from build123d import *

# Parameters (mm, degrees)
SKETCH_W      = 1500
SKETCH_H      = 400
PAD_DEPTH     = 500
SKETCH001_R   = 25
PAD001_DEPTH  = 150
SKETCH002_W   = 679.455933
SKETCH002_H   = 179.177673
SKETCH002_W_2 = 683.003968
SKETCH002_H_2 = 221.754555
POCKET_DEPTH  = 300


with BuildPart() as part:
    # Sketch → Pad (new body)
    with BuildSketch(Plane.XZ):
        with Locations((750, 200)):
            Rectangle(SKETCH_W, SKETCH_H)
    extrude(amount=PAD_DEPTH)

    # Sketch001 (on Face6 of Pad) → Pad001 (join)
    with BuildSketch(Plane.XZ.offset(500)):
        with Locations((45.287163, 361.134674)):
            Circle(SKETCH001_R)
        with Locations((49.395683, 36.55888)):
            Circle(SKETCH001_R)
        with Locations((1456.575439, 354.971802)):
            Circle(SKETCH001_R)
        with Locations((1452.466797, 32.450348)):
            Circle(SKETCH001_R)
    extrude(amount=PAD001_DEPTH)

    # Sketch002 (on Face1 of Pad001) → Pocket (cut)
    with BuildSketch(Plane(origin=(0, 0, 0), x_dir=(1, 0, 0), z_dir=(0, 0, -1))):
        with Locations((774.28888, 379.377991)):
            Rectangle(SKETCH002_W, SKETCH002_H)
        with Locations((772.514862, 148.753246)):
            Rectangle(SKETCH002_W_2, SKETCH002_H_2)
    extrude(amount=-POCKET_DEPTH, mode=Mode.SUBTRACT)


solid = part.part
Geometry check sheet. Reference: the model listing, model coordinates, mm. A direction names the side the tool comes from. Round coordinates to 2 decimals unless told otherwise and drop trailing zeros. Order: outer loops, then holes, each group sorted by start corner. A loop starts at its lowest first (then second) coordinate and runs counter-clockwise, first axis right, second up. Notation, with made-up numbers: M 87,-11 L 118,-11 A31 cw 118,21 Z; hole C 79.5,27 d6. An arc over 180 degrees is marked long. Answer in a Markdown table with one row per item. Add a question column.
Item 1: Set-up check for faces 1 (the face through (770, -381, 300)), 2 (the face through (1438.15, -573.95, 371.87)), 3 (the face through (0, -246, 197)): record each of +Z, -Z, +X, -X, +Y, -Y from which the full face is reachable in a straight line by a thin tool's end or side.
Item 2: Depth check by flat-ended pin: pin 1 Ø6 at (x, z) = (817.5, 117) entering from -Y. Enter the tip coordinate at first touch or a pass-through.
Item 3: Sectioned sample at A-A, the plane z = 245. Enter the section's corners in (x, y).
Item 4: Sectioned sample at D-D, the plane y = -578. Enter the section's corners in (x, z), plus the area to 3 significant figures.
Item 5: Draft check along Z on faces 4 (the face through (1114.017, -147, 148)), 5 (the face through (768, -150, 300)), 6 (the face through (73.24, -573.95, 44.07)). Enter one of: released by +Z, released by -Z, zero draft, split by the parting line, or undercut.
Item 6: Material ranges on L1, parallel to Y at x = 629.5, z = 261; L2, parallel to X at y = -400.5, z = 126; L3, parallel to Z at x = 556.5, y = -337, recorded low to high. Write a range as [from, to].
Item 7: Sectioned sample at B-B, the plane x = 613. Enter the section's corners in (y, z).
Item 8: Sectioned sample at C-C, the plane y = -110.5. Enter the section's corners in (x, z), plus the area to 3 significant figures.
Filled in:
| question | item | result |
|---|---|---|
| 1 | face 1 | -Z |
| 1 | face 2 | -Y |
| 1 | face 3 | +Z, -Z, -X, +Y, -Y |
| 2 | pin 1 | stops at y = -500 |
| 3 | outline | M 0,-500 L 1500,-500 L 1500,0 L 0,0 Z; hole M 431.01,-259.63 L 1114.02,-259.63 L 1114.02,-37.88 L 431.01,-37.88 Z; hole M 434.56,-468.97 L 1114.02,-468.97 L 1114.02,-289.79 L 434.56,-289.79 Z |
| 4 | outline | C 45.29,361.13 d50; C 49.4,36.56 d50; C 1452.47,32.45 d50; C 1456.58,354.97 d50 |
| 4 | area | 7,850 mm² |
| 5 | face 4 | zero draft |
| 5 | face 5 | released by -Z |
| 5 | face 6 | undercut |
| 6 | L1 | y = [-500, -468.97], [-289.79, -259.63], [-37.88, 0] |
| 6 | L2 | x = [0, 434.56], [1114.02, 1500] |
| 6 | L3 | z = [300, 400] |
| 7 | outline | M -500,0 L -468.97,0 L -468.97,300 L -289.79,300 L -289.79,0 L -259.63,0 L -259.63,300 L -37.88,300 L -37.88,0 L 0,0 L 0,400 L -500,400 Z |
| 8 | outline | M 0,0 L 431.01,0 L 431.01,300 L 1114.02,300 L 1114.02,0 L 1500,0 L 1500,400 L 0,400 Z |
| 8 | area | 395,000 mm² |
